Source: CAD feature listing. Evaluate the final solid. Frame: model axes, mm. Round coordinates to 2 decimals unless told otherwise and drop trailing zeros. Write each loop counter-clockwise with the first axis right and the second up, starting at its lowest first coordinate (ties: lowest second). Pieces come first, ordered by that corner, then holes. Notation, with made-up numbers: (-21.5, 52.25) -> (0.5, 52.25) arc R20 cw to (0.5, 61.25) -> close; hole circle Ø6 at (18.5, 24.5). An arc over 180 degrees is marked (long way). Put each result on its own line as item: value.
```python
from build123d import *

# Parameters (mm, degrees)
SKETCH1_W           = 1098.55
SKETCH1_H           = 50.8
BOSS_EXTRUDE1_DEPTH = 50.8
SKETCH2_W           = 44.45
SKETCH2_H           = 44.45
CUT_EXTRUDE1_DEPTH  = 1099.55
SKETCH5_R           = 3.302
SKETCH5_R_2         = 3.175
CUT_EXTRUDE2_DEPTH  = 50.8


with BuildPart() as part:
    # Sketch1 → Boss-Extrude1 (new body)
    with BuildSketch(Plane(origin=(0, 0, 0), x_dir=(0, 0, -1), z_dir=(1, 0, 0))):
        Rectangle(SKETCH1_W, SKETCH1_H)
    extrude(amount=BOSS_EXTRUDE1_DEPTH)

    # Sketch2 → Cut-Extrude1 (cut, through all)
    with BuildSketch(Plane.XY.offset(549.275)):
        with Locations((25.4, 0)):
            Rectangle(SKETCH2_W, SKETCH2_H)
    extrude(amount=-CUT_EXTRUDE1_DEPTH, mode=Mode.SUBTRACT)

    # Sketch5 → Cut-Extrude2 (cut)
    with BuildSketch(Plane(origin=(0, 25.4, 0), x_dir=(1, 0, 0), z_dir=(0, 1, 0))):
        with Locations((25.4, -346.075)):
            Circle(SKETCH5_R)
        with Locations((25.4, 0)):
            Circle(SKETCH5_R_2)
        with Locations((25.4, 346.075)):
            Circle(SKETCH5_R_2)
    extrude(amount=-CUT_EXTRUDE2_DEPTH, mode=Mode.SUBTRACT)


solid = part.part
```
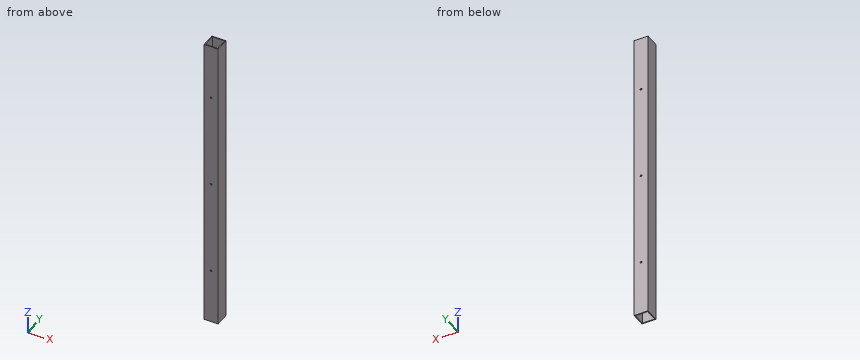
Q1. Cut plane A-A on y = 4. Output: boundary loops of the cut face in (x, z) (3 decimals).
Ans:
outline: (0, -549.275) -> (3.175, -549.275) -> (3.175, 549.275) -> (0, 549.275) -> close; (47.625, -549.275) -> (50.8, -549.275) -> (50.8, 549.275) -> (47.625, 549.275) -> close
Q2. Cut plane B-B on z = 268. Output: boundary loops of the cut face in (x, y) (3 decimals).
Ans:
outline: (0, -25.4) -> (50.8, -25.4) -> (50.8, 25.4) -> (0, 25.4) -> close; hole (3.175, -22.225) -> (47.625, -22.225) -> (47.625, 22.225) -> (3.175, 22.225) -> close
Q3. Material intervals for line 1 (Z direction, x = 25, y = 23) (3 decimals); line 2 (Z direction, x = 25.4, y = 24.65) (3 decimals); line 3 (X direction, y = -16, z = -305) (3 decimals), sorted ascending. Write a range as [from, to].
Ans:
line 1: z = [-549.275, -349.225], [-342.925, -3.15], [3.15, 342.797], [349.353, 549.275]
line 2: z = [-549.275, -349.25], [-342.9, -3.175], [3.175, 342.773], [349.377, 549.275]
line 3: x = [0, 3.175], [47.625, 50.8]
